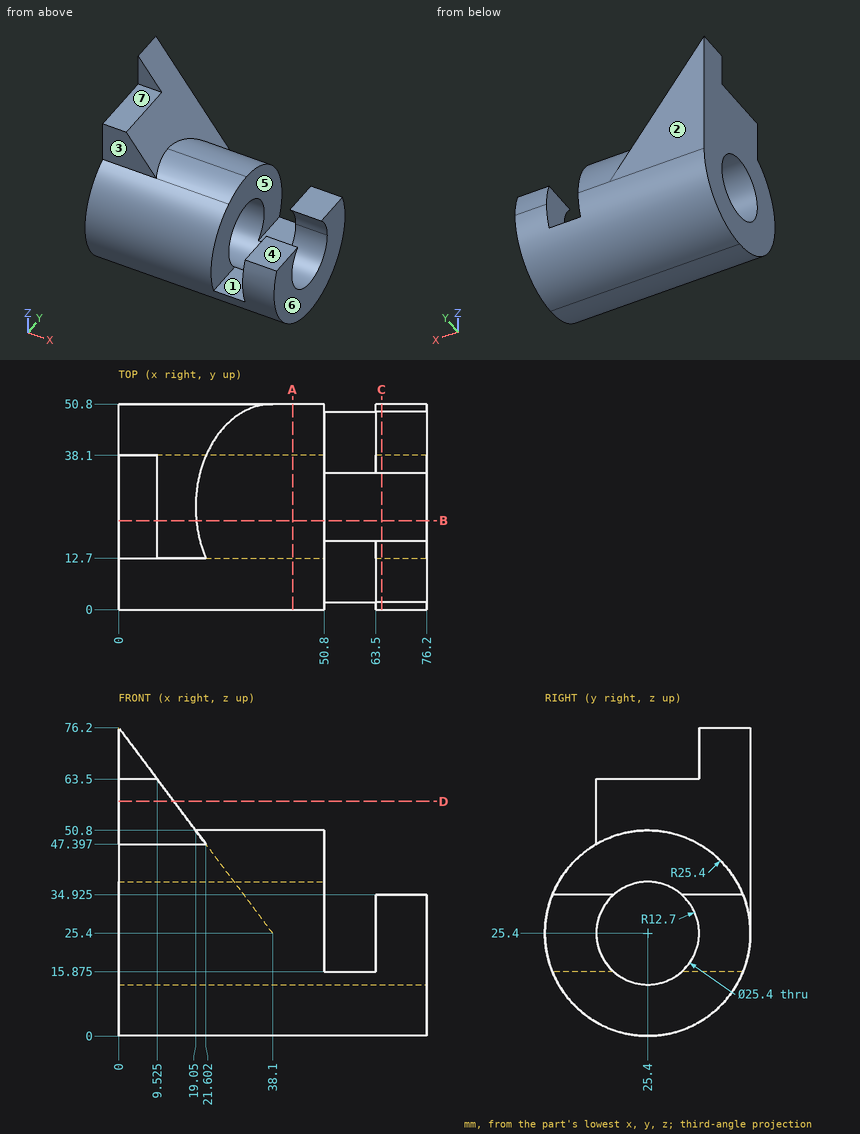
The drawing under review shows one solid part. Ordinate dimensions are in mm from its lowest x, y, z. A direction names the side the tool comes from. Round coordinates to 2 decimals unless told otherwise and drop trailing zeros. Loops run counter-clockwise (first coordinate to the right, second up) from the corner with the lowest first, then second, coordinate; pieces in that order, holes last. Notation, with made-up numbers: (-0.5, 28.25) - (32.5, 28.25) arc R29 ccw to (32.5, 57.25) - close; hole circle Ø7 at (56, 23.25). An arc over 180 degrees is marked (long way). One line per item, written item: value. Start each with the question number.
1) Insertion check: pin 1 Ø1.5 at (x, z) = (43, 29) entering from -Y; pin 2 Ø1.5 at (x, z) = (43, 47) entering from -Y; pin 3 Ø10 at (x, y) = (68.5, 7) entering from +Z (3 decimals). Each pin has a flat end and moves straight along its axis. Give the tip position at first contact, or say it passes through.
2) Consider section B-B on y = 22. Give the boundary of the cut face in (x, z) (1 decimal).
3) Consider section A-A on x = 43. Give the boundary of the cut face in (y, z).
4) For the marked faces 1, 2, 3 and 4, list the 3-axis set-ups (+Z, -Z, +X, -X, +Y, -Y) from which the entire face can be reached by the end or side of a thin tool; tool diameter is ignored.
5) Consider section C-C on x = 65. Give the boundary of the cut face in (y, z) (1 decimal).
6) Consider section D-D on z = 58. Give the boundary of the cut face in (x, y).
7) To check wall thickness, follow L1, parallel to Z at x = 44, y = 25; L2, parallel to Z at x = 59, y = 25.4; L3, parallel to Z at x = 23.5, y = 29.5. State the ranges of each line that lie inside material, in increasing order. Write a range as from..to.
8) Draft analysis for pull direction X (two halves, no side actions). For the marked faces 5, 6 and 7, state which applies: +X half, -X half, draft (parallel to the pull), parting line (faces both ways), or undercut.
Reported:
1. pin 1: stops at y = 0.16
1. pin 2: stops at y = 10.89
1. pin 3: stops at z = 34.925
2. outline: (0, 0.2) - (76.2, 0.2) - (76.2, 13.2) - (0, 13.2) - close; (0, 37.6) - (50.8, 37.6) - (50.8, 50.6) - (19.2, 50.6) - (9.5, 63.5) - (0, 63.5) - close
3. outline: circle Ø50.8 at (25.4, 25.4); hole circle Ø25.4 at (25.4, 25.4)
4. face 1: +Z, +Y, -Y
4. face 2: +Z, -Z, +X, -X, +Y
4. face 3: +Z, +X, -X, -Y
4. face 4: +Z, +X, +Y, -Y
5. outline: (1.9, 34.9) arc R25.4 ccw (long way) to (48.9, 34.9) - (33.8, 34.9) arc R12.7 cw (long way) to (17, 34.9) - close
6. outline: (0, 12.7) - (13.65, 12.7) - (13.65, 50.8) - (0, 50.8) - close
7. L1: z = 0..12.71, 38.09..50.8
7. L2: z = 0..12.7
7. L3: z = 0.33..13.38, 37.42..50.47
8. face 5: undercut
8. face 6: +X half
8. face 7: draft
